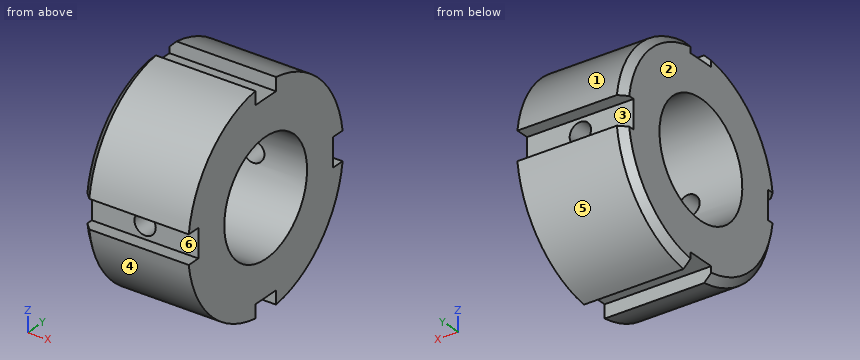
from build123d import *

# Parameters (mm, degrees)
SKETCH1_R               = 15
BOSS_EXTRUDE1_DEPTH     = 15
SKETCH2_R               = 8
CUT_EXTRUDE1_DEPTH      = 16
CHAMFER1_SIZE           = 1
SKETCH3_W               = 4
SKETCH3_H               = 4
CUT_EXTRUDE2_DEPTH      = 16
CIRPATTERN1_COUNT       = 4
SKETCH4_R               = 1.5
CUT_EXTRUDE4_DEPTH      = 18
CUT_EXTRUDE4_DEPTH_BACK = 15.866068747


with BuildPart() as part:
    # Sketch1 → Boss-Extrude1 (new body)
    with BuildSketch(Plane(origin=(0, 0, 0), x_dir=(0, 0, -1), z_dir=(1, 0, 0))):
        Circle(SKETCH1_R)
    extrude(amount=BOSS_EXTRUDE1_DEPTH)

    # Sketch2 → Cut-Extrude1 (cut, through all)
    with BuildSketch(Plane(origin=(15, 0, 0), x_dir=(0, 0, -1), z_dir=(1, 0, 0))):
        Circle(SKETCH2_R)
    extrude(amount=-CUT_EXTRUDE1_DEPTH, mode=Mode.SUBTRACT)

    # Chamfer1
    chamfer1_edges = [part.edges().sort_by_distance(p)[0] for p in [
        (0, 0, 15),
    ]]
    chamfer(chamfer1_edges, length=CHAMFER1_SIZE)

    # Sketch3 → Cut-Extrude2 (cut, through all)
    with BuildSketch(Plane(origin=(15, 0, 0), x_dir=(0, 0, -1), z_dir=(1, 0, 0))):
        with Locations((0, 15)):
            Rectangle(SKETCH3_W, SKETCH3_H)
    cut_extrude2 = extrude(amount=-CUT_EXTRUDE2_DEPTH, mode=Mode.SUBTRACT)

    # CirPattern1: Cut-Extrude2 ×4 about axis
    cirpattern1_axis = Axis((0, 0, 0), (1, 0, 0))
    for i in range(1, CIRPATTERN1_COUNT):
        add(cut_extrude2.rotate(cirpattern1_axis, i * 360 / CIRPATTERN1_COUNT), mode=Mode.SUBTRACT)

    # Sketch4 → Cut-Extrude4 (cut, two sides)
    with BuildSketch(Plane(origin=(0, 0, 0), x_dir=(1, 0, 0), z_dir=(0, 1, 0))) as cut_extrude4_sk:
        with Locations((7.5, 0)):
            Circle(SKETCH4_R)
    extrude(amount=CUT_EXTRUDE4_DEPTH, mode=Mode.SUBTRACT)
    extrude(cut_extrude4_sk.sketch, amount=-CUT_EXTRUDE4_DEPTH_BACK, mode=Mode.SUBTRACT)


solid = part.part
Can you work these out from the model? Positions are in its coordinate system, mm. Face numbers are marked on the shaded views. A direction names the side the tool comes from. Round coordinates to 2 decimals unless told otherwise and drop trailing zeros. Write each loop counter-clockwise with the first axis right and the second up, starting at its lowest first coordinate (ties: lowest second). Pieces come first, ordered by that corner, then holes. Notation, with made-up numbers: (26, 14.5) -> (59, 14.5) arc R3 ccw to (59, 18.5) -> close; hole circle Ø2 at (82.25, 9). An arc over 180 degrees is marked (long way). Use one line per item in the form item = value. Start each with the question number.
Q1. We'd pull the mould along Z, two halves only. Please class the marked faces 1, 2, 3 and 4: +Z half, -Z half, draft (parallel to the pull), parting line (faces both ways), or undercut.
Q2. Imagine slicing it at D-D (x = 7.5). Please give me the cut outline in (y, z).
Q3. If I drill on probe 1 along X at (y, z) = (9.7, 0); probe 2 along Y at (x, z) = (5.5, 0); probe 3 along Y at (x, z) = (1.25, -7.25), over which ranges is the centre line in solid material (lowest first)? Write a range as [from, to].
Q4. Which directions (+Z, -Z, +X, -X, +Y, -Y) give clear straight access to the entire face, cutting with the end or side of a thin tool? Please do the marked faces 5 and 6.
Q5. Imagine slicing it at B-B (y = 0). Please give me the cut outline in (x, z), then the cut area to 3 significant figures.
Q6. Imagine slicing it at C-C (x = 11.5). Please give me the cut outline in (y, z), then the cut area to 3 significant figures.
Q7. I'm going to push flat-ended pins straight in: P1, Ø1.5, axis at x = 4, z = -14, coming from the -Y side; P2, Ø1.2, axis at x = 5.5, y = -0.5, coming from the -Z side; P3, Ø1.5, axis at x = 5.5, y = -14.5, coming from the +Z side; P4, Ø5, axis at x = 7.5, z = 0, coming from the -Y side. Where does each tip first touch, or does it pass through?
Q8. Imagine slicing it at A-A (z = 0). Please give me the cut outline in (x, y).
Worked out:
q1.face_1 = +Z half
q1.face_2 = draft
q1.face_3 = undercut
q1.face_4 = -Z half
q2.outline = (-14.87, -2) arc R15 ccw to (-2, -14.87) -> (-2, -13) -> (2, -13) -> (2, -14.87) arc R15 ccw to (14.87, -2) -> (13, -2) -> (13, -1.5) -> (7.86, -1.5) arc R8 cw to (-7.86, -1.5) -> (-13, -1.5) -> (-13, -2) -> close; (-14.87, 2) -> (-13, 2) -> (-13, 1.5) -> (-7.86, 1.5) arc R8 cw to (7.86, 1.5) -> (13, 1.5) -> (13, 2) -> (14.87, 2) arc R15 ccw to (2, 14.87) -> (2, 13) -> (-2, 13) -> (-2, 14.87) arc R15 ccw to start
q3.probe_1 = [0, 6], [9, 15]
q3.probe_2 = [-13, -8], [8, 13]
q3.probe_3 = [-13.13, -3.38], [3.38, 13.13]
q4.face_5 = -Z, +X, -X, +Y
q4.face_6 = +X, -X, -Y
q5.outline = (0, -13) -> (15, -13) -> (15, -8) -> (0, -8) -> close; (0, 8) -> (15, 8) -> (15, 13) -> (0, 13) -> close
q5.area = 150 mm^2
q6.outline = (-14.87, -2) arc R15 ccw to (-2, -14.87) -> (-2, -13) -> (2, -13) -> (2, -14.87) arc R15 ccw to (14.87, -2) -> (13, -2) -> (13, 2) -> (14.87, 2) arc R15 ccw to (2, 14.87) -> (2, 13) -> (-2, 13) -> (-2, 14.87) arc R15 ccw to (-14.87, 2) -> (-13, 2) -> (-13, -2) -> close; hole circle Ø16 at (0, 0)
q6.area = 475 mm^2
q7.P1 = -7.03
q7.P2 = -13
q7.P3 = 5.99
q7.P4 = -14.87
q8.outline = (0, -13) -> (6, -13) -> (6, -8) -> (0, -8) -> close; (0, 8) -> (6, 8) -> (6, 13) -> (0, 13) -> close; (9, -13) -> (15, -13) -> (15, -8) -> (9, -8) -> close; (9, 8) -> (15, 8) -> (15, 13) -> (9, 13) -> close
